Autodesk Inventor part; units mm, degrees
ref_plane "YZ Plane" through (0, 0, 0) normal (1, 0, 0) x (0, 1, 0)
ref_plane "XZ Plane" through (0, 0, 0) normal (0, 1, 0) x (-1, 0, 0)
ref_plane "XY Plane" through (0, 0, 0) normal (0, 0, 1) x (1, 0, 0)
sketch "Sketch1" plane through (0, 0, 0) normal (0, 0, 1) x (1, 0, 0)
  line L0 (54, 22) -> (-54, 22)
  line L1 (-54, 22) -> (-54, -22)
  line L2 (-54, -22) -> (54, -22)
  line L3 (54, -22) -> (54, 22)
  line L4 (-54, 0) -> (54, 0) construction
  line L5 (0, 22) -> (0, -22) construction
  point P0 (0, 0)
  point P1 (0, 0)
  dimension "d0" = 108
  dimension "d1" = 44
extrude "Extrusion1" add sketch "Sketch1" along normal blind 25
fillet "Fillet1" radius 2 9 edges at (0, 22, 25) (0, -22, 25) (0, -22, 0) (0, 22, 0) (54, 0, 0) (54, 22, 12.5) (54, -22, 12.5) (-54, 0, 25) (-54, 0, 0)
sketch "Sketch2" plane through (54, -20, 2) normal (1, 0, 0) x (0, 0, -1)
  line L0 (0, 0) -> (-23, 0) construction
  line L1 (0, 40) -> (0, 0) construction
  line L2 (-23, 40) -> (0, 40) construction
  line L3 (-23, 0) -> (-23, 40) construction
  line L4 (-20, 18) -> (-10, 18)
  line L5 (-10, 18) -> (-10, 38)
  line L6 (-10, 38) -> (-20, 38)
  line L7 (-20, 38) -> (-20, 18)
  point P0 (2, 20)
  dimension "d5" = 10
  dimension "d6" = 20
  dimension "d7" = 3
  dimension "d8" = 18
extrude "Extrusion2" cut sketch "Sketch2" against normal blind 10
sketch "Sketch3" plane through (-54, -22, 23) normal (-1, 0, 0) x (0, 0, 1)
  line L0 (0, 44) -> (0, 0) construction
  line L1 (-21, 0) -> (0, 0) construction
  circle A0 centre (-5.5, 5.5) radius 2.5
  point P0 (-23, 22)
  dimension "d11" = 5
  dimension "d13" = 3
  dimension "d14" = 3
extrude "Extrusion3" add sketch "Sketch3" along normal blind 20
fillet "Fillet2" radius 2 3 edges at (53.4142, 21.4142, 24.4142) (53.4142, -21.4142, 24.4142) (54, 0, 25)
fillet "Fillet3" radius 5 1 edges at (49, -2, 22)
fillet "Fillet4" radius 5 3 edges at (49, 18, 22) (49, 18, 12) (49, -2, 12)
fillet "Fillet5" radius 2 6 edges at (-53.4142, 21.4142, 24.4142) (-53.4142, 21.4142, 0.5858) (-54, 22, 12.5) (-53.4142, -21.4142, 24.4142) (-53.4142, -21.4142, 0.5858) (-54, -22, 12.5)
properties part number "Transformer" material "PET Plastic"
Could you check a few things on this model? Use its own coordinates, in mm. A direction names the side the tool comes from. Coordinates: 2 decimals unless noted, no trailing zeros. Write each loop counter-clockwise with the first axis right and the second up, starting at its lowest first coordinate (ties: lowest second). Pieces come first, ordered by that corner, then holes. Notation, with made-up numbers: M -9.5,46 L 45.5,46 A16 cw 45.5,63 Z; hole C 20,35 d8. An arc over 180 degrees is marked long. One line per question, with ' | ' between items.
1) Imagine slicing it at A-A, the plane y = -9. Write out the boundary of the cut face in (x, z), and give its area (3 significant figures).
Checks:
outline: M -54,2 A2 ccw -52,0 L 52,0 A2 ccw 54,2 L 54,23 A2 ccw 52,25 L -52,25 A2 ccw -54,23 Z | area: 2,700 mm²
2) If we mould it in two halves opening along Y, with no side actions, what happens to faces 1 (the face through (-54, 0, 12)), 2 (the face through (49, 0, 13)), 3 (the face through (1, 22, 12))? For each: released by +Y, released by -Y, zero draft, split by the parting line, or undercut.
Checks:
face 1: zero draft | face 2: undercut | face 3: released by +Y
3) I need wall thicknesses on probe 1 along X at (y, z) = (-1.5, 3.25); probe 2 along X at (y, z) = (3.5, 12.75); probe 3 along Z at (x, y) = (-65, -17). Which ranges of each line are inside material? Lowest first, please. Write a range as [from, to].
Checks:
probe 1: [-54, 54] | probe 2: [-54, 44] | probe 3: [15.05, 19.95]
4) For pin 1 Ø3 at (y, z) = (10, 16) entering from +X; pin 2 Ø8 at (y, z) = (-10.5, 6.5) entering from -X, each with a flat end and sliding along its axis, tell me the tip position at first contact or that it passes through.
Checks:
pin 1: x = 44 | pin 2: x = -54
5) Imagine slicing it at C-C, the plane y = 11. Write out the boundary of the cut face in (x, z), and give its area (3 significant figures).
Checks:
outline: M -54,2 A2 ccw -52,0 L 52,0 A2 ccw 54,2 L 54,12 L 44,12 L 44,22 L 54,22 L 54,23 A2 ccw 52,25 L -52,25 A2 ccw -54,23 Z | area: 2,600 mm²
6) Imagine slicing it at D-D, the plane y = -16.5. Write out the boundary of the cut face in (x, z), and give its area (3 significant figures).
Checks:
outline: M -74,15 L -54,15 L -54,2 A2 ccw -52,0 L 52,0 A2 ccw 54,2 L 54,23 A2 ccw 52,25 L -52,25 A2 ccw -54,23 L -54,20 L -74,20 Z | area: 2,800 mm²
7) Imagine slicing it at B-B, the plane z = 9.5. Write out the boundary of the cut face in (x, y), and give its area (3 significant figures).
Checks:
outline: M -54,-20 A2 ccw -52,-22 L 52,-22 A2 ccw 54,-20 L 54,20 A2 ccw 52,22 L -52,22 A2 ccw -54,20 Z | area: 4,750 mm²
8) For faces 4 (the face through (-63.9, -16.6, 15)), 5 (the face through (49, 16, 21)), 6 (the face through (-1, 0, 0)), which set-ups out of +Z, -Z, +X, -X, +Y, -Y let a thin tool reach every point of the face, with its end or its side?
Checks:
face 4: -X | face 5: +X | face 6: -Z, +X, -X, +Y, -Y
